Check sheet for the modelled part. Datum: model origin and axes. Units: mm. Face numbers are marked on the shaded views. A direction names the side the tool comes from. Round coordinates to 2 decimals unless told otherwise and drop trailing zeros. Write each loop counter-clockwise with the first axis right and the second up, starting at its lowest first coordinate (ties: lowest second). Pieces come first, ordered by that corner, then holes.
Item 1: Section check A-A, the plane x = 10. Record the cut outline in (y, z).
Item 2: Set-up check for the marked faces 1 and 2: record each of +Z, -Z, +X, -X, +Y, -Y from which the full face is reachable in a straight line by a thin tool's end or side.
Item 3: Section check B-B, the plane y = 90. Record the cut outline in (x, z).
Item 4: Section check D-D, the plane z = -2. Record the cut outline in (x, y), plus the area to 3 significant figures.
Item 5: Depth check by flat-ended pin: pin 1 (3 mm diameter, centred on y = 58.5, z = -10.5, fed in from -X); pin 2 (5 mm diameter, centred on x = 8, y = 53.5, fed in from -Z); pin 3 (4 mm diameter, centred on y = 55.5, z = -14, fed in from +X). Enter the tip coordinate at first touch or a pass-through.
Item 6: Material ranges on line 1 along Y through (x, z) = (10, -0.8); line 2 along Y through (x, z) = (0.7, -10.5); line 3 along Z through (x, y) = (6.25, 13), recorded low to high.
Item 7: Section check C-C, the plane z = -10.5. Record the cut outline in (x, y).
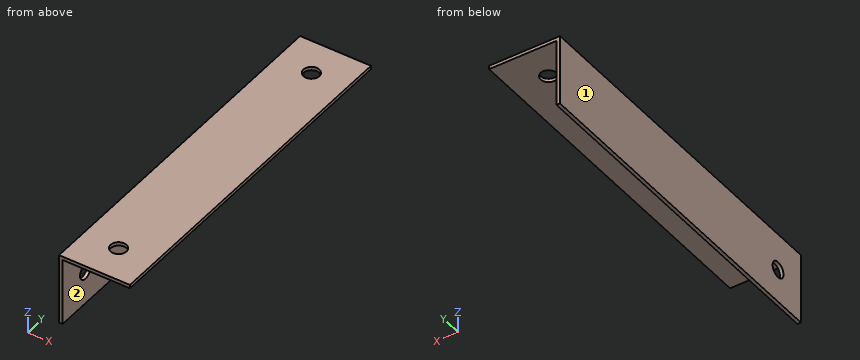
from build123d import *

# Parameters (mm, degrees)
EXTRUDE_1_DEPTH     = 100
SKETCH_2_R          = 2.25
CUT_EXTRUDE_1_DEPTH = 2
SKETCH_3_R          = 2.25
CUT_EXTRUDE_2_DEPTH = 2


with BuildPart() as part:
    # Эскиз1 → Бобышка-Вытянуть1 (new body)
    with BuildSketch(Plane(origin=(0, 0, 0), x_dir=(1, 0, 0), z_dir=(0, 1, 0))):
        Polygon((0, 0), (0, 20), (1, 20), (1, 1), (20, 1), (20, 0), align=None)
    extrude(amount=EXTRUDE_1_DEPTH)

    # Эскиз2 → Вырез-Вытянуть1 (cut, through all)
    with BuildSketch(Plane(origin=(0, 0, -1), x_dir=(-1, 0, 0), z_dir=(0, 0, -1))):
        with Locations((-10, 10)):
            Circle(SKETCH_2_R)
        with Locations((-10, 90)):
            Circle(SKETCH_2_R)
    extrude(amount=-CUT_EXTRUDE_1_DEPTH, mode=Mode.SUBTRACT)

    # Эскиз3 → Вырез-Вытянуть2 (cut, through all)
    with BuildSketch(Plane(origin=(1, 0, 0), x_dir=(0, 0, -1), z_dir=(1, 0, 0))):
        with Locations((10.5, 9.5)):
            Circle(SKETCH_3_R)
    extrude(amount=-CUT_EXTRUDE_2_DEPTH, mode=Mode.SUBTRACT)


solid = part.part
Values found:
1. outline: (0, -1) - (7.75, -1) - (7.75, 0) - (0, 0) - close; (12.25, -1) - (87.75, -1) - (87.75, 0) - (12.25, 0) - close; (92.25, -1) - (100, -1) - (100, 0) - (92.25, 0) - close
2. face 1: +Z, -Z, -X, +Y, -Y
2. face 2: -Z, +X, +Y, -Y
3. outline: (0, -20) - (1, -20) - (1, -1) - (7.75, -1) - (7.75, 0) - (0, 0) - close; (12.25, -1) - (20, -1) - (20, 0) - (12.25, 0) - close
4. outline: (0, 0) - (1, 0) - (1, 100) - (0, 100) - close
4. area: 100 mm2
5. pin 1: stops at x = 0
5. pin 2: stops at z = -1
5. pin 3: stops at x = 1
6. line 1: y = 0 to 7.75, 12.25 to 87.75, 92.25 to 100
6. line 2: y = 0 to 7.25, 11.75 to 100
6. line 3: z = -1 to 0
7. outline: (0, 0) - (1, 0) - (1, 7.25) - (0, 7.25) - close; (0, 11.75) - (1, 11.75) - (1, 100) - (0, 100) - close
